```python
from build123d import *

# Parameters (mm, degrees)
BOSS_EXTRUDE1_DEPTH = 37.6
SKETCH2_R           = 1.65
CUT_EXTRUDE1_DEPTH  = 69.530502022
SKETCH3_R           = 1.6
CUT_EXTRUDE2_DEPTH  = 69.260471168
FILLET1_R           = 18.8
FILLET2_R           = 2
FILLET3_R           = 4


with BuildPart() as part:
    # Sketch1 → Boss-Extrude1 (new body)
    with BuildSketch(Plane.XY):
        Polygon((-8.398458859, 29.360342427), (-6.398458859, 29.360342427), (-6.398458859, -8.239657573), (42.801541141, -8.239657573), (42.801541141, -10.239657573), (-8.398458859, -10.239657573), align=None)
    extrude(amount=BOSS_EXTRUDE1_DEPTH)

    # Sketch2 → Cut-Extrude1 (cut, through all)
    with BuildSketch(Plane(origin=(-6.398458859, 0, 0), x_dir=(0, 0, -1), z_dir=(1, 0, 0))):
        with Locations(Location((-34.3, 10.560342427, 0), (0, 0, 90))):
            Circle(SKETCH2_R)
        with Locations(Location((-26.55, 23.983736186, 0), (0, 0, 90))):
            Circle(SKETCH2_R)
        with Locations(Location((-11.05, 23.983736186, 0), (0, 0, 90))):
            Circle(SKETCH2_R)
        with Locations(Location((-3.3, 10.560342427, 0), (0, 0, 90))):
            Circle(SKETCH2_R)
        with Locations(Location((-11.05, -2.863051332, 0), (0, 0, 90))):
            Circle(SKETCH2_R)
        with Locations(Location((-26.55, -2.863051332, 0), (0, 0, 90))):
            Circle(SKETCH2_R)
        with BuildLine():
            Line((-12.2, 17.909663616), (-12.2, 3.909663616))
            ThreePointArc((-12.2, 3.909663616), (-18.8, -2.690336384), (-25.4, 3.909663616))
            Line((-25.4, 3.909663616), (-25.4, 17.909663616))
            ThreePointArc((-25.4, 17.909663616), (-18.8, 24.509663616), (-12.2, 17.909663616))
        make_face()
    extrude(amount=-CUT_EXTRUDE1_DEPTH, mode=Mode.SUBTRACT)

    # Sketch3 → Cut-Extrude2 (cut, through all)
    with BuildSketch(Plane(origin=(0, -8.239657573, 0), x_dir=(1, 0, 0), z_dir=(0, 1, 0))):
        with Locations(Location((0.001541141, -2.94858142, 0), (0, 0, 270))):
            Circle(SKETCH3_R)
        with Locations(Location((6.401541141, -2.94858142, 0), (0, 0, 270))):
            Circle(SKETCH3_R)
        with Locations(Location((12.801541141, -2.94858142, 0), (0, 0, 270))):
            Circle(SKETCH3_R)
        with Locations(Location((19.201541141, -2.94858142, 0), (0, 0, 270))):
            Circle(SKETCH3_R)
        with Locations(Location((25.601541141, -2.94858142, 0), (0, 0, 270))):
            Circle(SKETCH3_R)
        with Locations(Location((32.001541141, -2.94858142, 0), (0, 0, 270))):
            Circle(SKETCH3_R)
        with Locations(Location((38.401541141, -2.94858142, 0), (0, 0, 270))):
            Circle(SKETCH3_R)
        with Locations(Location((38.401541141, -34.14858142, 0), (0, 0, 90))):
            Circle(SKETCH3_R)
        with Locations(Location((32.001541141, -34.14858142, 0), (0, 0, 90))):
            Circle(SKETCH3_R)
        with Locations(Location((25.601541141, -34.14858142, 0), (0, 0, 90))):
            Circle(SKETCH3_R)
        with Locations(Location((19.201541141, -34.14858142, 0), (0, 0, 90))):
            Circle(SKETCH3_R)
        with Locations(Location((12.801541141, -34.14858142, 0), (0, 0, 90))):
            Circle(SKETCH3_R)
        with Locations(Location((6.401541141, -34.14858142, 0), (0, 0, 90))):
            Circle(SKETCH3_R)
        with Locations(Location((0.001541141, -34.14858142, 0), (0, 0, 90))):
            Circle(SKETCH3_R)
    extrude(amount=-CUT_EXTRUDE2_DEPTH, mode=Mode.SUBTRACT)

    # Fillet1
    fillet1_edges = [part.edges().sort_by_distance(p)[0] for p in [
        (-7.398458859, 29.360342427, 0),
        (-7.398458859, 29.360342427, 37.6),
    ]]
    fillet(fillet1_edges, radius=FILLET1_R - 0.0001)  # a hair under: the kernel refuses the full size

    # Fillet2
    fillet2_edges = [part.edges().sort_by_distance(p)[0] for p in [
        (-8.398458859, -10.239657573, 18.8),
    ]]
    fillet(fillet2_edges, radius=FILLET2_R)

    # Fillet3
    fillet3_edges = [part.edges().sort_by_distance(p)[0] for p in [
        (42.801541141, -9.239657573, 37.6),
        (42.801541141, -9.239657573, 0),
    ]]
    fillet(fillet3_edges, radius=FILLET3_R)


solid = part.part
```
Geometry check sheet. Reference: the model listing, model coordinates, mm. A direction names the side the tool comes from. Round coordinates to 2 decimals unless told otherwise and drop trailing zeros. Loops run counter-clockwise (first coordinate to the right, second up) from the corner with the lowest first, then second, coordinate; pieces in that order, holes last. Notation, with made-up numbers: (-26.75, -0.75) - (-3.75, -0.75) arc R24 ccw to (-3.75, 9.25) - close; hole circle Ø3 at (-32.75, -10.75). An arc over 180 degrees is marked (long way). Use a Markdown table: item, result.
Q1. Cross-section at A-A on z = 23.5. Record the cut outline in (x, y).
Solutions:
| item | result |
|---|---|
| outline | (-8.4, -8.24) arc R2 ccw to (-6.4, -10.24) - (42.8, -10.24) - (42.8, -8.24) - (-6.4, -8.24) - (-6.4, -0.72) - (-8.4, -0.72) - close; (-8.4, 22.54) - (-6.4, 22.54) - (-6.4, 28.76) - (-8.4, 28.76) - close |
Q2. Access from +Z, -Z, +X, -X, +Y, -Y to the whole of each face (thin tool, end or side, straight path). Record for faces 4 (the cylindrical face through (17.615, -9.226, 34.357)), 5 (the cylindrical face through (-7.384, 24.508, 18.945)).
Solutions:
| item | result |
|---|---|
| face 4 | +Y, -Y |
| face 5 | +X, -X |
Q3. Go/stop test with flat-tipped pins: P1, Ø4, axis at x = 38.4, z = 2.95, coming from the +Y side; P2, Ø3, axis at x = 6.4, z = 34.15, coming from the -Y side; P3, Ø3.5, axis at x = 12.8, z = 2.95, coming from the -Y side; P4, Ø4.5, axis at y = 23.98, z = 11.05, coming from the +X side. Record where each tip stops, or that it passes through.
Solutions:
| item | result |
|---|---|
| P1 | stops at y = -8.24 |
| P2 | passes through |
| P3 | stops at y = -10.24 |
| P4 | stops at x = -6.4 |
Q4. Cross-section at C-C on y = 20.5. Record the cut outline in (x, z).
Solutions:
| item | result |
|---|---|
| outline | (-8.4, 2.84) - (-6.4, 2.84) - (-6.4, 12.73) - (-8.4, 12.73) - close; (-8.4, 24.87) - (-6.4, 24.87) - (-6.4, 34.76) - (-8.4, 34.76) - close |
Q5. Cross-section at B-B on x = 12. Record the cut outline in (y, z), plus the area to 3 significant figures.
Solutions:
| item | result |
|---|---|
| outline | (-10.24, 0) - (-8.24, 0) - (-8.24, 1.56) - (-10.24, 1.56) - close; (-10.24, 4.33) - (-8.24, 4.33) - (-8.24, 32.76) - (-10.24, 32.76) - close; (-10.24, 35.53) - (-8.24, 35.53) - (-8.24, 37.6) - (-10.24, 37.6) - close |
| area | 64.1 mm2 |
Q6. Cross-section at D-D on z = 11.05. Record the cut outline in (x, y), plus the area to 3 significant figures.
Solutions:
| item | result |
|---|---|
| outline | (-8.4, -8.24) arc R2 ccw to (-6.4, -10.24) - (42.8, -10.24) - (42.8, -8.24) - (-6.4, -8.24) - (-6.4, -4.51) - (-8.4, -4.51) - close; (-8.4, -1.21) - (-6.4, -1.21) - (-6.4, 22.33) - (-8.4, 22.33) - close; (-8.4, 25.63) - (-6.4, 25.63) - (-6.4, 27.69) - (-8.4, 27.69) - close |
| area | 160 mm2 |
Q7. Material ranges on line 1 (Y direction, x = 38, z = 8); line 2 (X direction, y = 7.5, z = 25.5), recorded low to high.
Solutions:
| item | result |
|---|---|
| line 1 | y = -10.24 to -8.24 |
| line 2 | x = -8.4 to -6.4 |
Q8. Draft check along X on faces 1 (the cylindrical face through (11.72, -9.23, 35.33)), 2 (the flat face through (-6.398, 7, 27)), 3 (the cylindrical face through (-7.38, -3.22, 24.94)). Enter one of: released by +X, released by -X, zero draft, split by the parting line, or undercut.
Solutions:
| item | result |
|---|---|
| face 1 | undercut |
| face 2 | released by +X |
| face 3 | zero draft |
